Autodesk Inventor part; units mm, degrees
ref_plane "YZ Plane" through (0, 0, 0) normal (1, 0, 0) x (0, 1, 0)
ref_plane "XZ Plane" through (0, 0, 0) normal (0, 1, 0) x (-1, 0, 0)
ref_plane "XY Plane" through (0, 0, 0) normal (0, 0, 1) x (1, 0, 0)
sketch "Эскиз1" plane through (0, 0, 0) normal (0, 0, 1) x (1, 0, 0)
  circle A0 centre (0, 0) radius 7.95
  circle A1 centre (0, 0) radius 11
  circle A2 centre (0, 0) radius 6
  dimension "d0" = 15.9
  dimension "d1" = 22
  dimension "d2" = 12
extrude "Выдавливание1" add sketch "Эскиз1" against normal blind 2.5 contours A0
extrude "Выдавливание2" add sketch "Эскиз1" along normal blind 9.7 contours A0 | A1
sketch "Эскиз2" plane through (0, 0, 0) normal (0, 0, -1) x (-1, 0, 0)
  circle A0 centre (3.6709, -8.2173) radius 1.5
  circle A1 centre (-3.6709, 8.2173) radius 1.5
  circle A2 centre (3.6709, -8.2173) radius 1.5
  circle A3 centre (-3.6709, 8.2173) radius 1.5
  point P0 (0, 0)
  dimension "d7" = 3
  dimension "d8" = 3
extrude "Выдавливание3" cut sketch "Эскиз2" along normal mid plane 30
properties part number "factory barrier adapter"
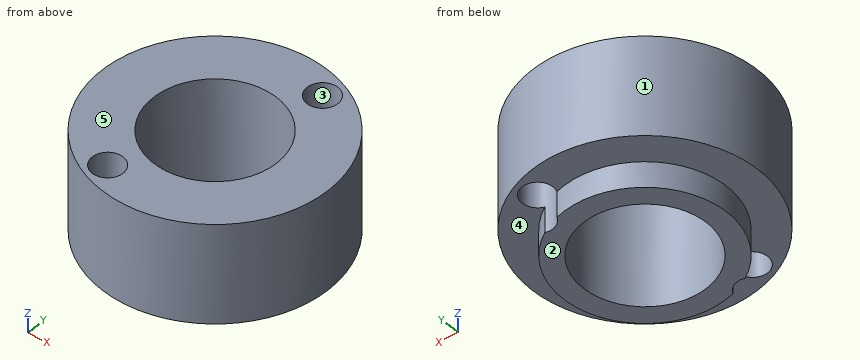
Part model, mm, in its own coordinate system. Face numbers are marked on the shaded views. A direction names the side the tool comes from. Coordinates: 2 decimals unless noted, no trailing zeros. Loops run counter-clockwise (first coordinate to the right, second up) from the corner with the lowest first, then second, coordinate; pieces in that order, holes last. Notation, with made-up numbers: (-0.75, 89) - (15.25, 89) arc R20 cw to (15.25, 103) - close; hole circle Ø6 at (-11.75, 30). An arc over 180 degrees is marked (long way). Write each question's results on one line, items separated by ' | '. Start each with the question number.
Q1. Which spindle directions (+Z, -Z, +X, -X, +Y, -Y) get a long thin tool onto all of the face, cutting with end or side? Do the marked faces 4 and 5. Say none if no direction does.
Q2. Slice it at D-D on z = -1.5. Give the cut face in (x, y).
Q3. Slice it at A-A on y = 0. Give the cut face in (x, z), and give its area (3 significant figures).
Q4. Two-plate mould, pull along X, no slides. Class the marked faces 1, 2 and 3: +X half, -X half, draft (parallel to the pull), parting line (faces both ways), or undercut.
Q5. Slice it at C-C on x = -4.5. Give the cut face in (y, z).
Q6. Drop flat-ended pins along their axis: pin 1 Ø2.5 at (x, y) = (-3.67, -8.22) entering from +Z; pin 2 Ø4 at (y, z) = (5, 6) entering from -X; pin 3 Ø1 at (y, z) = (8, 4) entering from +X. Give the stop position or say it passes through.
Q7. Probe line 1 along Y through (x, z) = (-3, 5.5); line 2 along Y through (x, z) = (-0.25, 1.5); line 3 along X through (y, z) = (4.25, 3.75). List the from-to ranges inside material, lowest first.
Answer:
1) face 4: -Z | face 5: +Z, +X, -X, +Y, -Y
2) outline: (-4.13, -6.79) arc R1.5 cw to (-2.3, -7.61) arc R7.95 ccw to (4.13, 6.79) arc R1.5 cw to (2.3, 7.61) arc R7.95 ccw to start; hole circle Ø12 at (0, 0)
3) outline: (-11, 0) - (-7.95, 0) - (-7.95, -2.5) - (-6, -2.5) - (-6, 9.7) - (-11, 9.7) - close; (6, -2.5) - (7.95, -2.5) - (7.95, 0) - (11, 0) - (11, 9.7) - (6, 9.7) - close | area: 107 mm2
4) face 1: parting line | face 2: draft | face 3: undercut
5) outline: (-10.04, 0) - (-9.47, 0) - (-9.47, 9.7) - (-10.04, 9.7) - close; (-6.97, 0) - (-6.55, 0) - (-6.55, -2.5) - (-3.97, -2.5) - (-3.97, 9.7) - (-6.97, 9.7) - close; (3.97, -2.5) - (6.55, -2.5) - (6.55, 0) - (10.04, 0) - (10.04, 9.7) - (3.97, 9.7) - close
6) pin 1: passes through | pin 2: stops at x = -10.58 | pin 3: stops at x = 8.05
7) line 1: y = -10.58 to -9.56, -6.88 to -5.2, 5.2 to 10.58 | line 2: y = -11 to -5.99, 5.99 to 11 | line 3: x = -10.15 to -4.24, 4.24 to 10.15
